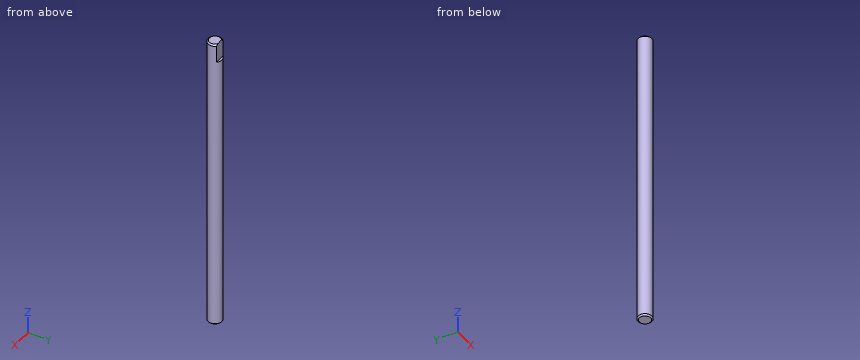
Autodesk Inventor part; units mm, degrees
ref_plane "YZ Plane" through (0, 0, 0) normal (1, 0, 0) x (0, 1, 0)
ref_plane "XZ Plane" through (0, 0, 0) normal (0, 1, 0) x (-1, 0, 0)
ref_plane "XY Plane" through (0, 0, 0) normal (0, 0, 1) x (1, 0, 0)
sketch "Sketch1" plane through (0, 0, 0) normal (0, 0, 1) x (1, 0, 0)
  circle A0 centre (0, 0) radius 3
  dimension "d0" = 6
extrude "Extrusion1" add sketch "Sketch1" along normal blind 130
thread "Thread1"
chamfer "Chamfer1" distance 0.6 angle 45 1 edges at (-3, 0, 130)
chamfer "Chamfer2" distance 0.6 angle 45 1 edges at (-3, 0, 0)
sketch "Sketch2" plane through (0, 0, 130) normal (0, 0, 1) x (1, 0, 0)
  line L0 (3.8696, 4.6025) -> (-3.8038, 4.6025)
  line L1 (-3.8038, 4.6025) -> (-3.8038, 2)
  line L2 (-3.8038, 2) -> (3.8696, 2)
  line L3 (3.8696, 2) -> (3.8696, 4.6025)
  point P0 (0, 0)
  dimension "d11" = 2
extrude "Extrusion2" cut sketch "Sketch2" against normal blind 8
properties part number "popychacz"
Input: part model. Units: mm. Frame: model coordinates. Give positions to 0.01 mm unless a question says otherwise; leave off trailing zeros. Loops run counter-clockwise (first coordinate to the right, second up) from the corner with the lowest first, then second, coordinate; pieces in that order, holes last. Notation, with made-up numbers: (8, 27) -> (53, 27) arc R15 cw to (53, 54) -> close; hole circle Ø8 at (-15.5, 4). An arc over 180 degrees is marked (long way). Answer as a JSON object with one key per item and string values. Group by question number.
Item 1: Cut plane A-A, the plane z = 81. Return the cut outline in (x, y).
Item 2: Pin query (flat end, axial travel): P1, Ø2, axis at x = -2, z = 46.5, coming from the +Y side; P2, Ø1.3, axis at x = 0, z = 126, coming from the +Y side; P3, Ø1, axis at y = 1.5, z = 19, coming from the +X side. Return the tip coordinate at first contact, or that it passes through.
Item 3: Line query: probe 1 along Y at (x, z) = (-2, 88); probe 2 along Y at (x, z) = (0.35, 60); probe 3 along X at (y, z) = (-0.1, 89.5). Output: solid intervals per line, ascending.
Checks:
{
 "1": {"outline": "circle Ø6 at (0, 0)"},
 "2": {"P1": "stops at y = 2.83", "P2": "stops at y = 2", "P3": "stops at x = 2.83"},
 "3": {"probe 1": "y = -2.24 to 2.24", "probe 2": "y = -2.98 to 2.98", "probe 3": "x = -3 to 3"}
}
